Part model, mm, in its own coordinate system. Face numbers are marked on the shaded views. A direction names the side the tool comes from. Give positions to 0.01 mm unless a question says otherwise; leave off trailing zeros. Write each loop counter-clockwise with the first axis right and the second up, starting at its lowest first coordinate (ties: lowest second). Pieces come first, ordered by that corner, then holes. Notation, with made-up numbers: M 75,38.5 L 95,38.5 A26 cw 95,52.5 Z; hole C 51,81 d5. An arc over 180 degrees is marked long. Use CSV: the item, a comma, the result in double quotes. Start each with the question number.
Item 1: Which spindle directions (+Z, -Z, +X, -X, +Y, -Y) get a long thin tool onto all of the face, cutting with end or side? Do the marked faces 5, 6 and 7. Say none if no direction does.
Item 2: Pin check, flat tips, straight feed: pin 1 (10 mm diameter, centred on x = 6.5, y = 6.5, fed in from -Z); pin 2 (10 mm diameter, centred on x = 15.5, y = 15, fed in from +Z); pin 3 (10 mm diameter, centred on x = 28.5, y = 10.5, fed in from +Z); pin 4 (1 mm diameter, centred on x = 35.5, z = 11, fed in from -Y). Stop position of each tip, or through.
Item 3: Mould opens along Y. For the marked faces 1, 2, 3 and 4 say: released by +Y, released by -Y, zero draft, split by the parting line, or undercut.
Item 4: Cut at B-B (x = 23.8). List the corners of the cut face in (y, z), then the cut area to 3 significant figures.
Item 5: Drill centre lines: line 1 (Y direction, x = 23.8, z = 2); line 2 (X direction, y = 10, z = 2.5); line 3 (X direction, y = 10, z = 7.25). Where is each one in solid material? Low to high. Write a range as [from, to].
Item 6: Cut at C-C (z = 3). List the corners of the cut face in (x, y), then the cut area to 3 significant figures.
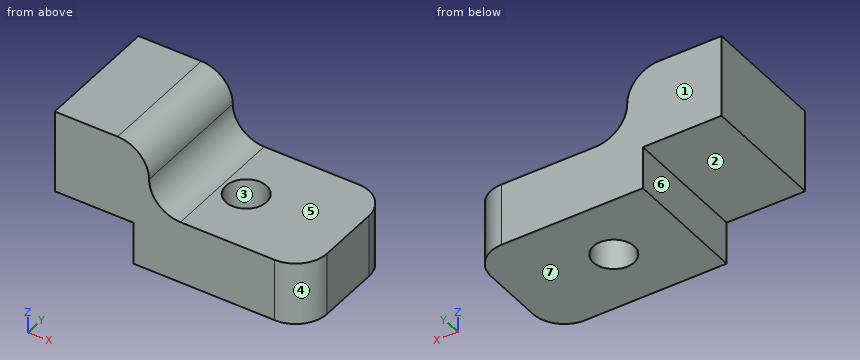
Autodesk Fusion 360 part; units mm, degrees
sketch "Sketch1" plane through (0, 0, 0) normal (0, 0, 1) x (1, 0, 0)
  line L0 (0, 0) -> (40, 0)
  line L1 (40, 0) -> (40, 20)
  line L2 (40, 20) -> (0, 20)
  line L3 (0, 20) -> (0, 0)
  dimension "d1" = 40
  dimension "d2" = 20
extrude "Extrude1" add sketch "Sketch1" along normal blind 20
sketch "Sketch2" plane through (0, 0, 0) normal (0, 0, -1) x (1, 0, 0)
  line L0 (0, 0) -> (0, -20)
  line L1 (0, -20) -> (40, -20)
  line L2 (40, -20) -> (40, 0)
  line L3 (40, 0) -> (0, 0)
  line L4 (0, 0) -> (10, 0)
  line L5 (10, 0) -> (10, -20)
  line L6 (10, -20) -> (0, -20)
  line L7 (0, -20) -> (0, 0)
  line L8 (10, -10) -> (23.8, -10)
  circle A0 centre (23.8, -10) radius 3.25
  dimension "d5" = 10
  dimension "d6" = 20
  dimension "d7" = 13.8
  dimension "d8" = 6.5
extrude "Extrude2" cut sketch "Sketch2" against normal blind 7.8 contours L0 L1 L3 L4 L5 L6 L7 | A0
extrude "Extrude3" cut 1 faces at (24.5115, 8.6722, 7.8) along direction (0, 0, 1) blind 210
sketch "Sketch3" plane through (0, 0, 20) normal (0, 0, 1) x (-1, 0, 0)
  circle A0 centre (-23.8, -10) radius 3.25
  line L0 (0, -20) -> (0, 0)
  line L1 (0, 0) -> (-40, 0)
  line L2 (-40, 0) -> (-40, -20)
  line L3 (-40, -20) -> (0, -20)
  line L4 (-40, -20) -> (-15, -20)
  line L5 (-15, -20) -> (-15, 0)
  line L6 (-15, 0) -> (-40, 0)
  line L7 (-40, 0) -> (-40, -20)
  dimension "d13" = 25
  dimension "d14" = 20
extrude "Extrude4" cut sketch "Sketch3" against normal blind 10 contours L1 L2 L3 L4 L5 L6 L7
fillet "Fillet1" radius 5 2 edges at (15, 10, 10) (15, 10, 20)
fillet "Fillet2" radius 5 2 edges at (40, 0, 5) (40, 20, 5)
sketch "Sketch4" plane through (0, 0, 0) normal (0, 1, 0) x (1, 0, 0)
extrude "Extrude5" cut 1 faces at (10, 6.6667, 2.6) along direction (1, 0, 0) blind 0.5
extrude "Extrude6" add 1 faces at (10.5, 6.6667, 2.6) along direction (-1, 0, 0) blind 0.5
sketch "Sketch5" plane through (0, 0, 20) normal (0, 0, 1) x (-1, 0, 0)
  line L0 (-10, 0) -> (-10, -20)
  line L1 (-10, -20) -> (0, -20)
  line L2 (0, -20) -> (0, 0)
  line L3 (0, 0) -> (-10, 0)
sketch "Sketch6" plane through (0, 0, 0) normal (0, -1, 0) x (1, 0, 0)
  line L0 (10, 0) -> (35, 0)
  line L1 (35, 0) -> (35, 10)
  line L2 (35, 10) -> (20, 10)
  arc A0 (15, 15) -> (20, 10) centre (20, 15) ccw
  arc A1 (15, 15) -> (10, 20) centre (10, 15) ccw
  line L3 (10, 20) -> (0, 20)
  line L4 (0, 20) -> (0, 7.8)
  line L5 (0, 7.8) -> (10, 7.8)
  line L6 (10, 7.8) -> (10, 0)
sketch "Sketch7" plane through (0, 0, 0) normal (0, -1, 0) x (1, 0, 0)
sketch "Sketch8" plane through (0, 0, 10) normal (0, 0, 1) x (-1, 0, 0)
  arc A0 (-40, -15) -> (-35, -20) centre (-35, -15) ccw
  line L0 (-35, -20) -> (-20, -20)
  line L1 (-20, -20) -> (-20, 0)
  line L2 (-20, 0) -> (-35, 0)
  arc A1 (-35, 0) -> (-40, -5) centre (-35, -5) ccw
  line L3 (-40, -5) -> (-40, -15)
  circle A2 centre (-23.8, -10) radius 3.25
extrude "Extrude7" cut 1 faces at (10, 6.6667, 2.6) along direction (1, 0, 0) blind 2.5
extrude "Extrude8" add 1 faces at (4.1667, 6.6667, 7.8) along direction (0, 0, -1) blind 1
Worked answers:
1,face 5,"+Z, +X, +Y, -Y"
1,face 6,"-Z, -X, +Y, -Y"
1,face 7,"-Z, +X, -X, +Y, -Y"
2,pin 1,"stops at z = 6.8"
2,pin 2,"stops at z = 19.98"
2,pin 3,"stops at z = 10"
2,pin 4,"passes through"
3,face 1,"released by +Y"
3,face 2,"zero draft"
3,face 3,"undercut"
3,face 4,"released by -Y"
4,outline,"M 0,0 L 6.75,0 L 6.75,10 L 0,10 Z; M 13.25,0 L 20,0 L 20,10 L 13.25,10 Z"
4,area,"135 mm^2"
5,line 1,"y = [0, 6.75], [13.25, 20]"
5,line 2,"x = [12.5, 20.55], [27.05, 40]"
5,line 3,"x = [0, 20.55], [27.05, 40]"
6,outline,"M 12.5,0 L 35,0 A5 ccw 40,5 L 40,15 A5 ccw 35,20 L 12.5,20 Z; hole C 23.8,10 d6.5"
6,area,"506 mm^2"
